Answer from the drawing. Dimensions are ordinates in mm from the lowest x, y and z of the part. Coordinates: 2 decimals unless noted, no trailing zeros. Write each loop counter-clockwise with the first axis right and the second up, starting at its lowest first coordinate (ties: lowest second). Pieces come first, ordered by that corner, then holes.
(1) The part is cut by section C-C on z = 24.5. Determine the outline of the cut face in (x, y) (3 decimals), plus the area to 3 significant figures.
(2) For a pull along Y with two mould halves and no side action, classify the marked faces 1, 2 and 3 as +Y half, -Y half, draft (parallel to the pull), parting line (faces both ways), or undercut.
(3) Given P1, Ø5, axis at x = 3.5, z = 60.5, coming from the +Y side; P2, Ø4, axis at y = 86, z = 46, coming from the -X side; P3, Ø1.5, axis at x = 6, y = 40.5, coming from the +Z side; P4, Ø1, axis at x = 6.5, z = 54, coming from the +Y side, each flat-ended and moving along its own axis, determine where each tip first touches the part or whether it passes through.
(4) The part is cut by section A-A on z = 46. Determine the outline of the cut face in (x, y), plus the area to 3 significant figures.
(5) The part is cut by section B-B on y = 46. Determine the outline of the cut face in (x, z).
(6) Straight lines are drawn through the part: line 1 (Z direction, x = 7.5, y = 46); line 2 (Y direction, x = 6, z = 13); line 3 (Z direction, x = 9.25, y = 40). For each, find the intervals that lie inside material, in ascending order.
(7) The part is cut by section D-D on y = 26. Determine the outline of the cut face in (x, z), plus the area to 3 significant figures.
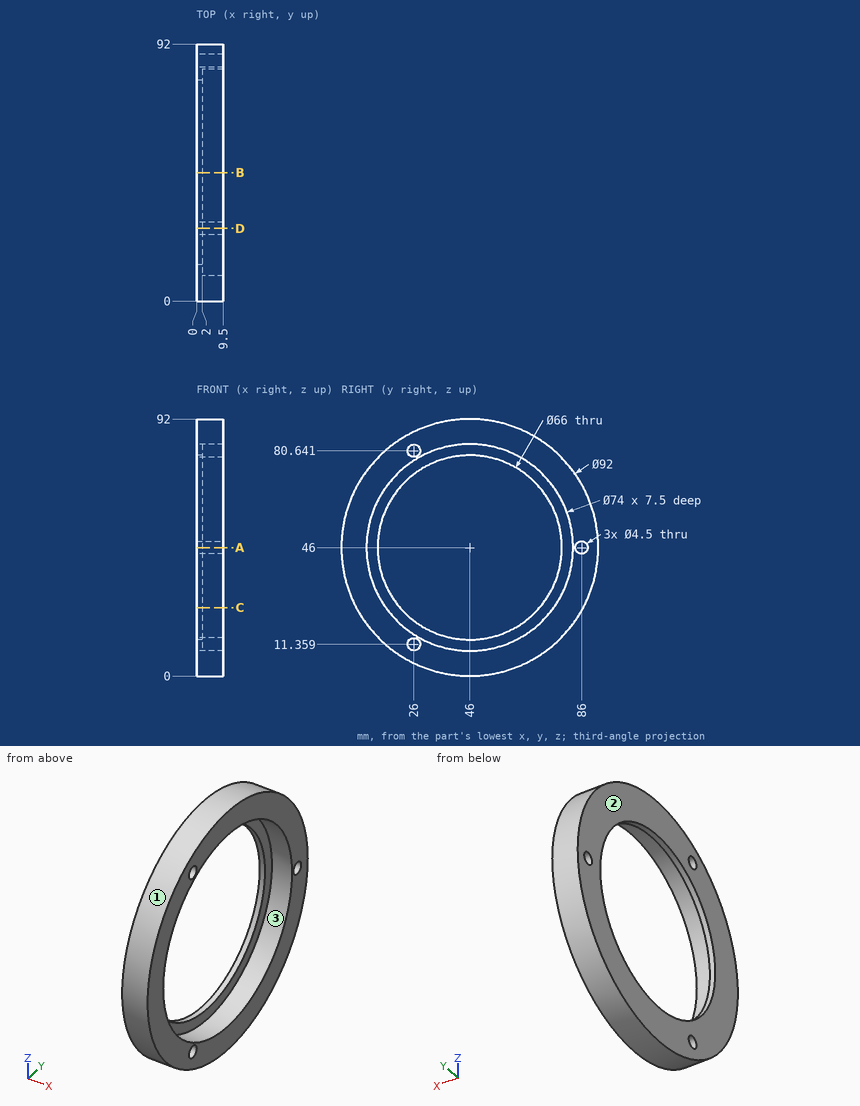
Model answer:
1. outline: (0, 5.334) - (9.5, 5.334) - (9.5, 15.888) - (2, 15.888) - (2, 20.965) - (0, 20.965) - close; (0, 71.035) - (2, 71.035) - (2, 76.112) - (9.5, 76.112) - (9.5, 86.666) - (0, 86.666) - close
1. area: 221 mm2
2. face 1: parting line
2. face 2: draft
2. face 3: undercut
3. P1: stops at y = 90.41
3. P2: passes through
3. P3: stops at z = 91.75
3. P4: stops at y = 91.38
4. outline: (0, 0) - (9.5, 0) - (9.5, 9) - (2, 9) - (2, 13) - (0, 13) - close; (0, 79) - (2, 79) - (2, 83) - (9.5, 83) - (9.5, 83.75) - (0, 83.75) - close; (0, 88.25) - (9.5, 88.25) - (9.5, 92) - (0, 92) - close
4. area: 144 mm2
5. outline: (0, 0) - (9.5, 0) - (9.5, 9) - (2, 9) - (2, 13) - (0, 13) - close; (0, 79) - (2, 79) - (2, 83) - (9.5, 83) - (9.5, 92) - (0, 92) - close
6. line 1: z = 0 to 9, 83 to 92
6. line 2: y = 13.95 to 24.46, 27.54 to 29.27, 62.73 to 78.05
6. line 3: z = 0.39 to 9.49, 82.51 to 91.61
7. outline: (0, 4.58) - (9.5, 4.58) - (9.5, 9.11) - (0, 9.11) - close; (0, 13.61) - (9.5, 13.61) - (9.5, 14.87) - (2, 14.87) - (2, 19.75) - (0, 19.75) - close; (0, 72.25) - (2, 72.25) - (2, 77.13) - (9.5, 77.13) - (9.5, 78.39) - (0, 78.39) - close; (0, 82.89) - (9.5, 82.89) - (9.5, 87.42) - (0, 87.42) - close
7. area: 130 mm2
